Drawing for the job (mm, zero at the part's lowest x, y, z). A direction names the side the tool comes from. Round coordinates to 2 decimals unless told otherwise and drop trailing zeros. Write each loop counter-clockwise with the first axis right and the second up, starting at its lowest first coordinate (ties: lowest second). Pieces come first, ordered by that corner, then holes.
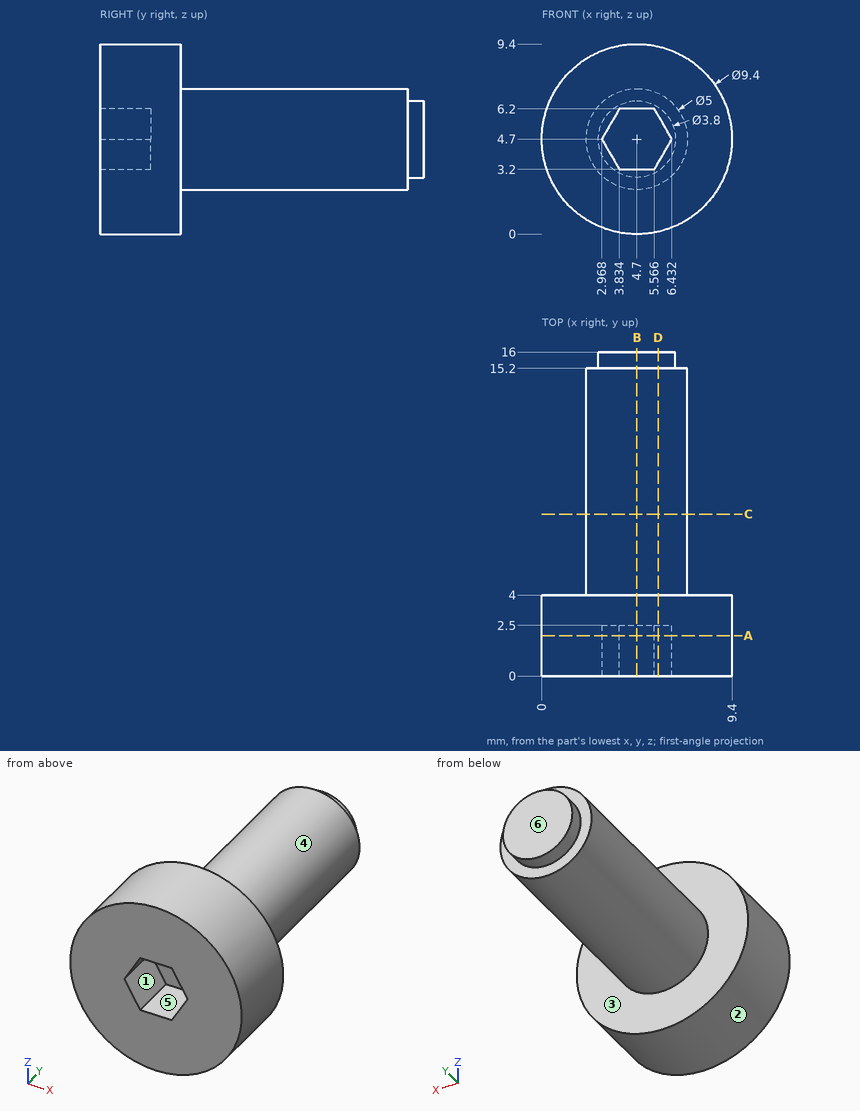
Q1. Saw through at A-A, the plane y = 2. Write the cut outline in (x, z).
Q2. Two-plate mould, pull along X, no slides. Class the marked faces 4, 5 and 6: released by +X, released by -X, zero draft, split by the parting line, or undercut.
Q3. Saw through at C-C, the plane y = 8. Write the cut outline in (x, z), and give its area (3 significant figures).
Q4. Saw through at D-D, the plane x = 5.75. Write the cut outline in (y, z), and give its area (3 significant figures).
Q5. Saw through at B-B, the plane x = 4.7. Write the cut outline in (y, z), and give its area (3 significant figures).
Q6. Drop flat-ended pins along their axis: P1, Ø5, axis at x = 7.5, y = 5.5, coming from the -Z side; P2, Ø1.5, axis at x = 1.5, z = 2, coming from the +Y side; P3, Ø0.9, axis at x = 4.5, z = 5, coming from the -Y side. Give the stop position or say it passes through.
Q7. Tool access for the marked faces 1, 2 and 3: list every direction of +Z, -Z, +X, -X, +Y, -Y with a clear straight run to the whole face (end or side of a thin tool).
Q8. Wall check: line 1 (Y direction, x = 1.25, z = 6); line 2 (Y direction, x = 3.75, z = 3.75); line 3 (Z direction, x = 5, y = 2). Give the ranges that are in metal, low to high.
Computed:
1. outline: circle Ø9.4 at (4.7, 4.7); hole (2.97, 4.7) - (3.83, 3.2) - (5.57, 3.2) - (6.43, 4.7) - (5.57, 6.2) - (3.83, 6.2) - close
2. face 4: split by the parting line
2. face 5: undercut
2. face 6: zero draft
3. outline: circle Ø5 at (4.7, 4.7)
3. area: 19.6 mm2
4. outline: (0, 0.12) - (4, 0.12) - (4, 2.43) - (15.2, 2.43) - (15.2, 3.12) - (16, 3.12) - (16, 6.28) - (15.2, 6.28) - (15.2, 6.97) - (4, 6.97) - (4, 9.28) - (0, 9.28) - (0, 5.88) - (2.5, 5.88) - (2.5, 3.52) - (0, 3.52) - close
4. area: 84.1 mm2
5. outline: (0, 0) - (4, 0) - (4, 2.2) - (15.2, 2.2) - (15.2, 2.8) - (16, 2.8) - (16, 6.6) - (15.2, 6.6) - (15.2, 7.2) - (4, 7.2) - (4, 9.4) - (0, 9.4) - (0, 6.2) - (2.5, 6.2) - (2.5, 3.2) - (0, 3.2) - close
5. area: 89.1 mm2
6. P1: stops at z = 0.07
6. P2: stops at y = 4
6. P3: stops at y = 2.5
7. face 1: -Y
7. face 2: +Y, -Y
7. face 3: +Y
8. line 1: y = 0 to 4
8. line 2: y = 2.5 to 16
8. line 3: z = 0.01 to 3.2, 6.2 to 9.39
